```python
from build123d import *

# Parameters (mm, degrees)
SKETCH1_W           = 20
SKETCH1_H           = 4
BOSS_EXTRUDE1_DEPTH = 30
SKETCH2_W           = 40
SKETCH2_H           = 40
BOSS_EXTRUDE2_DEPTH = 20
FILLET1_R           = 10


with BuildPart() as part:
    # Sketch1 → Boss-Extrude1 (new body)
    with BuildSketch(Plane.XY):
        with Locations((-20, -2)):
            Rectangle(SKETCH1_W, SKETCH1_H)
    extrude(amount=BOSS_EXTRUDE1_DEPTH)

    # Sketch2 → Boss-Extrude2 (add)
    with BuildSketch(Plane.XY):
        with Locations((-10, 16)):
            Rectangle(SKETCH2_W, SKETCH2_H)
    extrude(amount=-BOSS_EXTRUDE2_DEPTH)

    # Fillet1
    # the kernel refuses this fillet: 10 mm, written as the material it adds along each edge
    with BuildSketch(Plane(origin=(-10, 0, 0), x_dir=(0, 1, 0), z_dir=(-1, 0, 0))) as fillet1_piece_1:
        with BuildLine():
            CenterArc((FILLET1_R, -FILLET1_R), FILLET1_R, 90, 90)
            Line((0, -FILLET1_R), (0, 0))
            Line((0, 0), (FILLET1_R, 0))
        make_face()
    extrude(amount=20)
    # the kernel refuses this fillet: 10 mm, written as the material it takes off along each edge
    with BuildSketch(Plane(origin=(10, 36, 25), x_dir=(-1, 0, 0), z_dir=(0, 0, -1))) as fillet1_2_piece_1:
        with BuildLine():
            CenterArc((FILLET1_R, -FILLET1_R), FILLET1_R, 90, 90)
            Line((0, -FILLET1_R), (0, 0))
            Line((0, 0), (FILLET1_R, 0))
        make_face()
    extrude(amount=70, mode=Mode.SUBTRACT)
    with BuildSketch(Plane(origin=(10, 0, 30), x_dir=(0, 0, -1), z_dir=(-1, 0, 0))) as fillet1_2_piece_2:
        with BuildLine():
            CenterArc((8, 10), FILLET1_R, 216.869897646, 53.130102354)
            Line((0, 4), (0, 0))
            Line((0, 0), (8, 0))
        make_face()
    extrude(amount=60, mode=Mode.SUBTRACT)


solid = part.part
```
Could you check a few things on this model? Use its own coordinates, in mm. A direction names the side the tool comes from. Round coordinates to 2 decimals unless told otherwise and drop trailing zeros. Write each loop counter-clockwise with the first axis right and the second up, starting at its lowest first coordinate (ties: lowest second). Pieces come first, ordered by that corner, then holes. Notation, with made-up numbers: M -38.5,8 L -12.5,8 A15 cw -12.5,13 Z; hole C -28,11.5 d9. An arc over 180 degrees is marked long. Write each question's results on one line, items separated by ' | '. Start each with the question number.
1. Imagine slicing it at C-C on z = 24. List the corners of the cut face in (x, y) for me.
2. Imagine slicing it at B-B on y = 4. List the corners of the cut face in (x, z) for me, and give its area (3 significant figures).
3. I'm going to push flat-ended pins straight in: pin 1 Ø11 at (y, z) = (4, 17.5) entering from +X; pin 2 Ø2 at (x, y) = (5.5, 31.5) entering from +Z; pin 3 Ø13 at (x, z) = (-19.5, 17) entering from +Y. Where does each tip first touch, or does it pass through?
4. On a 3-axis mill with a long thin cutter (end or side, diameter ignored), from which of +Z, -Z, +X, -X, +Y, -Y can I reach the whole of each face in a straight line? I mean faces 1 (the face through (-20, 0, 16)), 2 (the face through (-10, -2, 12)), 3 (the face through (6.99, 33.15, -9.86)), 4 (the face through (-15, -4, 0)), 5 (the face through (-10, 21, 0)). Say none if no direction works.
5. Imagine slicing it at D-D on y = 23. List the corners of the cut face in (x, z) for me, and give its area (3 significant figures).
6. Imagine slicing it at A-A on x = -19.5. List the corners of the cut face in (y, z) for me, and give its area (3 significant figures).
7. I need wall thicknesses on L1, parallel to Z at x = -20, y = 15.5; L2, parallel to Y at x = -14, z = 20.5; L3, parallel to Z at x = -24, y = 3.5. Which ranges of each line are inside material? Lowest first, please. Write a range as from..to.
Result sheet:
1) outline: M -30,-4 L -10,-4 L -10,-0.2 L -30,-0.2 Z
2) outline: M -30,-20 L 10,-20 L 10,0 L -10,0 L -10,2 L -30,2 Z | area: 840 mm^2
3) pin 1: stops at x = -10 | pin 2: stops at z = 0 | pin 3: stops at y = 0
4) face 1: +Z, +X, -X, +Y | face 2: +Z, +X, +Y, -Y | face 3: +Z, -Z, +X, +Y | face 4: +Z, -Z, +X, -X, -Y | face 5: +Z, +X, +Y
5) outline: M -30,-20 L 10,-20 L 10,0 L -30,0 Z | area: 800 mm^2
6) outline: M -4,-20 L 36,-20 L 36,0 L 10,0 A10 cw 0,10 L 0,22 A10 ccw -4,30 Z | area: 932 mm^2
7) L1: z = -20..0 | L2: y = -4..0 | L3: z = -20..2.4
